Could you check a few things on this model? Use its own coordinates, in mm. A direction names the side the tool comes from. Give positions to 0.01 mm unless a question says otherwise; leave off trailing zeros. Write each loop counter-clockwise with the first axis right and the second up, starting at its lowest first coordinate (ties: lowest second). Pieces come first, ordered by that corner, then holes. Notation, with made-up numbers: (73.25, 74) - (109.25, 74) arc R33 cw to (109.25, 105) - close; hole circle Ø10 at (29.5, 23). An arc over 180 degrees is marked (long way). Answer as CSV lines item,"result". Start each with the question number.
Q1. Will these pins go through, and if not, where does the flat tip stop? pin 1 Ø10 at (x, y) = (-63.5, -2.5) entering from +Z; pin 2 Ø3.5 at (x, y) = (-33.73, -1.13) entering from -Z; pin 3 Ø2 at (y, z) = (13.87, 20.1) entering from -X.
Q2. Imagine slicing it at B-B on z = 3. List the corners of the cut face in (x, y) for me.
Q3. Imagine slicing it at C-C on y = 7. List the corners of the cut face in (x, z) for me, and give its area (3 significant figures).
Q4. On a 3-axis mill with a long thin cutter (end or side, diameter ignored), from which of +Z, -Z, +X, -X, +Y, -Y can I reach the whole of each face in a straight line? I mean faces 4 (the face through (-36, -5.5, 16)), 5 (the face through (-42.045, -7.086, 16.628)), 6 (the face through (-34, 10, 6.7)), 7 (the face through (-34.34, 23.97, 12.44)), 8 (the face through (-32.567, 14, 10)). Say none if no direction works.
Q5. If I drill on line 1 along Z through (x, y) = (-31.4, 3.87); line 2 along Y through (x, z) = (-51, 6); line 3 along Z through (x, y) = (-47, 7), over which ranges is the centre line in solid material (lowest first)?
Q6. Imagine slicing it at D-D on z = 17.5. List the corners of the cut face in (x, y) for me.
Q7. Imagine slicing it at A-A on x = -52. List the corners of the cut face in (y, z) for me.
Q8. We'd pull the mould along Y, two halves only. Please class faces 1 (the face through (-31.071, -4.074, 15.968)), 2 (the face through (-29.567, 13, 15)), 3 (the face through (-32.567, 14, 20)): pulls with the +Y half, pulls with the -Y half, needs draft (parallel to the pull), parting line crosses it, or undercut.
```python
from build123d import *

# Parameters (mm, degrees)
SKETCH_1_R                = 1.5
SKETCH_1_R_2              = 6.25
EXTRUDE_1_DEPTH           = 25.5
SKETCH_2_R                = 18.5
CUT_EXTRUDE_1_DEPTH       = 17.5
SKETCH_3_W                = 9.3
SKETCH_3_H                = 31.5
CUT_EXTRUDE_2_DEPTH       = 6.7
FILLET_1_R                = 20
SKETCH_4_R                = 1.5
CUT_EXTRUDE_3_DEPTH       = 44.630787393
FILLET_3_R                = 2
FILLET_4_R                = 2
FILLET_5_R                = 5
SKETCH_5_R                = 6
CUT_EXTRUDE_4_DEPTH       = 4
SKETCH_6_R                = 1.3
CUT_EXTRUDE_5_DEPTH       = 3
MOVE_BODY_1_OUTLINE_R     = 1.5
MOVE_BODY_1_OUTLINE_R_2   = 6.25
MOVE_BODY_1_DEPTH         = 25.5
MOVE_START                = 6.7
MOVE_BODY_1_2_OUTLINE_R   = 1.5
MOVE_BODY_1_2_OUTLINE_R_2 = 18.5
MOVE_BODY_1_2_DEPTH       = 18.8
MOVE_BODY_1_3_OUTLINE_R   = 1.5
MOVE_BODY_1_3_OUTLINE_R_2 = 6.25
MOVE_BODY_1_3_DEPTH       = 8
MOVE_START_2              = -29.5669682
MOVE_BODY_1_4_OUTLINE_W   = 31.5
MOVE_BODY_1_4_OUTLINE_H   = 18.8
MOVE_BODY_1_4_DEPTH       = 9.2969682
MOVE_START_3              = -32.5669682
MOVE_BODY_1_5_OUTLINE_R   = 1.3
MOVE_BODY_1_5_DEPTH       = 3
MOVE_START_4              = -21
MOVE_BODY_1_6_DEPTH       = 47
MOVE_START_5              = 22
MOVE_BODY_1_7_OUTLINE_R   = 6
MOVE_BODY_1_7_DEPTH       = 4


with BuildPart() as part:
    # 草图1 → 凸台-拉伸1 (new body)
    with BuildSketch(Plane.XY):
        with BuildLine():
            Line((21, 0), (21, 26))
            Line((21, 26), (-29.5669682, 26))
            Line((-29.5669682, 26), (-29.5669682, -5.5))
            Line((-29.5669682, -5.5), (-20.2669682, -5.5))
            ThreePointArc((-20.2669682, -5.5), (2.774316836, -20.815935388), (21, 0))
        make_face()
        with Locations((15.5, 0)):
            Circle(SKETCH_1_R, mode=Mode.SUBTRACT)
        with Locations((-15.5, 0)):
            Circle(SKETCH_1_R, mode=Mode.SUBTRACT)
        with Locations((-7.75, 13.423393759)):
            Circle(SKETCH_1_R, mode=Mode.SUBTRACT)
        with Locations((7.75, 13.423393759)):
            Circle(SKETCH_1_R, mode=Mode.SUBTRACT)
        with Locations((7.75, -13.423393759)):
            Circle(SKETCH_1_R, mode=Mode.SUBTRACT)
        with Locations((-7.75, -13.423393759)):
            Circle(SKETCH_1_R, mode=Mode.SUBTRACT)
        with Locations((0, 7)):
            Circle(SKETCH_1_R_2, mode=Mode.SUBTRACT)
    extrude(amount=EXTRUDE_1_DEPTH)

    # 草图2 → 切除-拉伸1 (cut)
    with BuildSketch(Plane.XY.offset(25.5)):
        Circle(SKETCH_2_R)
    extrude(amount=-CUT_EXTRUDE_1_DEPTH, mode=Mode.SUBTRACT)

    # 草图3 → 切除-拉伸2 (cut)
    with BuildSketch(Plane(origin=(0, 0, 0), x_dir=(-1, 0, 0), z_dir=(0, 0, -1))):
        with Locations((24.92, 10.25)):
            Rectangle(SKETCH_3_W, SKETCH_3_H)
    extrude(amount=-CUT_EXTRUDE_2_DEPTH, mode=Mode.SUBTRACT)

    # 圆角1
    fillet_1_edges = [part.edges().sort_by_distance(p)[0] for p in [
        (21, 26, 12.75),
    ]]
    fillet(fillet_1_edges, radius=FILLET_1_R)

    # 草图4 → 切除-拉伸3 (cut, through all)
    with BuildSketch(Plane(origin=(0, 0, 6.7), x_dir=(-1, 0, 0), z_dir=(0, 0, -1))):
        with Locations((25.407304845, 18.87)):
            Circle(SKETCH_4_R)
        with Locations((25.407304845, -1.13)):
            Circle(SKETCH_4_R)
    extrude(amount=-CUT_EXTRUDE_3_DEPTH, mode=Mode.SUBTRACT)

    # 圆角3
    fillet_3_edges = [part.edges().sort_by_distance(p)[0] for p in [
        (-29.5669682, 10.25, 25.5),
    ]]
    fillet(fillet_3_edges, radius=FILLET_3_R)

    # 圆角4
    fillet_4_edges = [part.edges().sort_by_distance(p)[0] for p in [
        (-20.2669682, -5.5, 12.75),
    ]]
    fillet(fillet_4_edges, radius=FILLET_4_R)

    # 圆角5
    # the kernel refuses this fillet: 5 mm, written as the material it takes off along each edge
    with BuildSketch(Plane(origin=(-29.5669682, -5.5, -5.8), x_dir=(1, 0, 0), z_dir=(0, 0, 1))) as fillet_5_piece_1:
        with BuildLine():
            CenterArc((FILLET_5_R, FILLET_5_R), FILLET_5_R, 180, 90)
            Line((0, FILLET_5_R), (0, 0))
            Line((0, 0), (FILLET_5_R, 0))
        make_face()
    extrude(amount=41.8, mode=Mode.SUBTRACT)

    # 草图5 → 切除-拉伸4 (cut)
    with BuildSketch(Plane(origin=(0, 26, 0), x_dir=(1, 0, 0), z_dir=(0, 1, 0))):
        with Locations(Location((-21.5669682, -17.5, 0), (0, 0, 270))):
            Circle(SKETCH_5_R)
    extrude(amount=-CUT_EXTRUDE_4_DEPTH, mode=Mode.SUBTRACT)

    # 草图6 → 切除-拉伸5 (cut)
    with BuildSketch(Plane.ZY.offset(29.5669682)):
        with Locations(Location((20.1, 13.87, 0), (0, 0, 270))):
            Circle(SKETCH_6_R)
        with Locations(Location((20.1, 3.87, 0), (0, 0, 270))):
            Circle(SKETCH_6_R)
        with Locations(Location((10.1, 3.87, 0), (0, 0, 270))):
            Circle(SKETCH_6_R)
        with Locations(Location((10.1, 13.87, 0), (0, 0, 270))):
            Circle(SKETCH_6_R)
    extrude(amount=-CUT_EXTRUDE_5_DEPTH, mode=Mode.SUBTRACT)

    # Move Body 1: read off the stored shape, not the designer's step
    # Move Body 1 outline → Move Body 1 (cut)
    with BuildSketch(Plane.XY):
        with BuildLine():
            Line((1, 26), (-20.27, 26))
            Line((-20.27, 26), (-20.27, 22))
            Line((-20.27, 22), (-20.27, -6.146923411))
            ThreePointArc((-20.27, -6.146923411), (-20.024941251, -6.475836873), (-19.852135348, -6.847826087))
            ThreePointArc((-19.852135348, -6.847826087), (3.471682423, -20.711045873), (21, 0))
            Line((21, 0), (21, 6))
            ThreePointArc((21, 6), (15.142135624, 20.142135624), (1, 26))
        make_face()
        with Locations((7.75, 13.423393759)):
            Circle(MOVE_BODY_1_OUTLINE_R, mode=Mode.SUBTRACT)
        with Locations((-7.75, -13.423393759)):
            Circle(MOVE_BODY_1_OUTLINE_R, mode=Mode.SUBTRACT)
        with Locations((7.75, -13.423393759)):
            Circle(MOVE_BODY_1_OUTLINE_R, mode=Mode.SUBTRACT)
        with Locations((-15.5, 0)):
            Circle(MOVE_BODY_1_OUTLINE_R, mode=Mode.SUBTRACT)
        with Locations((15.5, 0)):
            Circle(MOVE_BODY_1_OUTLINE_R, mode=Mode.SUBTRACT)
        with Locations((-7.75, 13.423393759)):
            Circle(MOVE_BODY_1_OUTLINE_R, mode=Mode.SUBTRACT)
        with Locations((0, 7)):
            Circle(MOVE_BODY_1_OUTLINE_R_2, mode=Mode.SUBTRACT)
    extrude(amount=MOVE_BODY_1_DEPTH, mode=Mode.SUBTRACT)

    # Move Body 1 2 outline → Move Body 1 2 (add)
    with BuildSketch(Plane.XY.offset(MOVE_START)):
        with BuildLine():
            Line((-20.27, 26), (-60.133936399, 26))
            ThreePointArc((-60.133936399, 26), (-74.276072023, 20.142135624), (-80.133936399, 6))
            Line((-80.133936399, 6), (-80.133936399, 0))
            ThreePointArc((-80.133936399, 0), (-62.605618822, -20.711045873), (-39.281801051, -6.847826087))
            ThreePointArc((-39.281801051, -6.847826087), (-38.552080618, -5.871450365), (-37.391121494, -5.5))
            Line((-37.391121494, -5.5), (-34.5669682, -5.5))
            ThreePointArc((-34.5669682, -5.5), (-31.031434294, -4.035533906), (-29.5669682, -0.5))
            ThreePointArc((-29.5669682, -0.5), (-28.102502106, -4.035533905), (-24.5669682, -5.5))
            Line((-24.5669682, -5.5), (-21.742814905, -5.5))
            ThreePointArc((-21.742814905, -5.5), (-20.938499413, -5.668859211), (-20.27, -6.146923411))
            Line((-20.27, -6.146923411), (-20.27, 22))
            Line((-20.27, 22), (-20.27, 26))
        make_face()
        with Locations((-33.726631554, -1.13)):
            Circle(MOVE_BODY_1_2_OUTLINE_R, mode=Mode.SUBTRACT)
        with Locations((-25.407304845, -1.13)):
            Circle(MOVE_BODY_1_2_OUTLINE_R, mode=Mode.SUBTRACT)
        with Locations((-33.726631554, 18.87)):
            Circle(MOVE_BODY_1_2_OUTLINE_R, mode=Mode.SUBTRACT)
        with Locations((-25.407304845, 18.87)):
            Circle(MOVE_BODY_1_2_OUTLINE_R, mode=Mode.SUBTRACT)
        with Locations((-59.133936399, 0)):
            Circle(MOVE_BODY_1_2_OUTLINE_R_2, mode=Mode.SUBTRACT)
    extrude(amount=MOVE_BODY_1_2_DEPTH)

    # Move Body 1 3 outline → Move Body 1 3 (add)
    with BuildSketch(Plane.XY):
        with BuildLine():
            Line((-38.863936399, 22), (-38.863936399, 26))
            Line((-38.863936399, 26), (-60.133936399, 26))
            ThreePointArc((-60.133936399, 26), (-74.276072023, 20.142135624), (-80.133936399, 6))
            Line((-80.133936399, 6), (-80.133936399, 0))
            ThreePointArc((-80.133936399, 0), (-62.605618822, -20.711045873), (-39.281801051, -6.847826087))
            ThreePointArc((-39.281801051, -6.847826087), (-39.108995148, -6.475836873), (-38.863936399, -6.146923411))
            Line((-38.863936399, -6.146923411), (-38.863936399, 22))
        make_face()
        with Locations((-51.383936399, 13.423393759)):
            Circle(MOVE_BODY_1_3_OUTLINE_R, mode=Mode.SUBTRACT)
        with Locations((-66.883936399, -13.423393759)):
            Circle(MOVE_BODY_1_3_OUTLINE_R, mode=Mode.SUBTRACT)
        with Locations((-51.383936399, -13.423393759)):
            Circle(MOVE_BODY_1_3_OUTLINE_R, mode=Mode.SUBTRACT)
        with Locations((-74.633936399, 0)):
            Circle(MOVE_BODY_1_3_OUTLINE_R, mode=Mode.SUBTRACT)
        with Locations((-43.633936399, 0)):
            Circle(MOVE_BODY_1_3_OUTLINE_R, mode=Mode.SUBTRACT)
        with Locations((-59.133936399, 7)):
            Circle(MOVE_BODY_1_3_OUTLINE_R_2, mode=Mode.SUBTRACT)
        with Locations((-66.883936399, 13.423393759)):
            Circle(MOVE_BODY_1_3_OUTLINE_R, mode=Mode.SUBTRACT)
    extrude(amount=MOVE_BODY_1_3_DEPTH)

    # Move Body 1 4 outline → Move Body 1 4 (cut)
    with BuildSketch(Plane.YZ.offset(MOVE_START_2)):
        with Locations((10.25, 16.1)):
            Rectangle(MOVE_BODY_1_4_OUTLINE_W, MOVE_BODY_1_4_OUTLINE_H)
    extrude(amount=MOVE_BODY_1_4_DEPTH, mode=Mode.SUBTRACT)

    # Move Body 1 5 outline → Move Body 1 5 (cut)
    with BuildSketch(Plane.YZ.offset(MOVE_START_3)):
        with Locations((13.87, 20.1)):
            Circle(MOVE_BODY_1_5_OUTLINE_R)
        with Locations((3.87, 20.1)):
            Circle(MOVE_BODY_1_5_OUTLINE_R)
        with Locations((3.87, 10.1)):
            Circle(MOVE_BODY_1_5_OUTLINE_R)
        with Locations((13.87, 10.1)):
            Circle(MOVE_BODY_1_5_OUTLINE_R)
    extrude(amount=MOVE_BODY_1_5_DEPTH, mode=Mode.SUBTRACT)

    # Move Body 1 6 outline → Move Body 1 6 (cut)
    with BuildSketch(Plane(origin=(0, 0, 0), x_dir=(1, 0, 0), z_dir=(0, 1, 0)).offset(MOVE_START_4)):
        with BuildLine():
            ThreePointArc((-29.5669682, -23.5), (-30.152754638, -24.914213563), (-31.5669682, -25.5))
            Line((-31.5669682, -25.5), (-20.27, -25.5))
            Line((-20.27, -25.5), (-20.27, -6.7))
            Line((-20.27, -6.7), (-29.566968204, -6.7))
            Line((-29.566968204, -6.7), (-29.5669682, -23.5))
        make_face()
    extrude(amount=MOVE_BODY_1_6_DEPTH, mode=Mode.SUBTRACT)

    # Move Body 1 7 outline → Move Body 1 7 (cut)
    with BuildSketch(Plane(origin=(0, 0, 0), x_dir=(1, 0, 0), z_dir=(0, 1, 0)).offset(MOVE_START_5)):
        with Locations((-37.5669682, -17.5)):
            Circle(MOVE_BODY_1_7_OUTLINE_R)
    extrude(amount=MOVE_BODY_1_7_DEPTH, mode=Mode.SUBTRACT)


solid = part.part
```
Conclusion:
1,pin 1,"z = 8"
1,pin 2,"z = 6.7"
1,pin 3,"x = -78.92"
2,outline,"(-80.13, 0) arc R21 ccw to (-39.28, -6.85) arc R2 cw to (-38.86, -6.15) - (-38.86, 26) - (-60.13, 26) arc R20 ccw to (-80.13, 6) - close; hole circle Ø3 at (-74.63, 0); hole circle Ø3 at (-66.88, -13.42); hole circle Ø3 at (-66.88, 13.42); hole circle Ø12.5 at (-59.13, 7); hole circle Ø3 at (-51.38, -13.42); hole circle Ø3 at (-51.38, 13.42); hole circle Ø3 at (-43.63, 0)"
3,outline,"(-80.11, 0) - (-65.38, 0) - (-65.38, 8) - (-76.26, 8) - (-76.26, 25.5) - (-80.11, 25.5) - close; (-52.88, 0) - (-38.86, 0) - (-38.86, 6.7) - (-29.57, 6.7) - (-29.57, 23.5) arc R2 ccw to (-31.57, 25.5) - (-42.01, 25.5) - (-42.01, 8) - (-52.88, 8) - close"
3,area,"526 mm^2"
4,face 4,"+Z, -Z, +X, -Y"
4,face 5,"+Z"
4,face 6,"-Z, +X, +Y, -Y"
4,face 7,"+Y"
4,face 8,"+X"
5,line 1,"6.7 to 8.8, 11.4 to 18.8, 21.4 to 25.49"
5,line 2,"-19.36 to -14.87, -11.97 to 11.97, 14.87 to 26"
5,line 3,"0 to 8"
6,outline,"(-80.13, 0) arc R21 ccw to (-39.28, -6.85) arc R2 cw to (-37.39, -5.5) - (-34.57, -5.5) arc R5 ccw to (-29.57, -0.5) - (-29.57, 26) - (-31.57, 26) - (-31.57, 22) - (-43.57, 22) - (-43.57, 26) - (-60.13, 26) arc R20 ccw to (-80.13, 6) - close; hole circle Ø37 at (-59.13, 0); hole circle Ø3 at (-33.73, -1.13); hole circle Ø3 at (-33.73, 18.87)"
7,outline,"(-19.75, 0) - (-14.79, 0) - (-14.79, 8) - (-17.07, 8) - (-17.07, 25.5) - (-19.75, 25.5) - close; (-12.06, 0) - (12.06, 0) - (12.06, 8) - (-12.06, 8) - close; (14.79, 0) - (26, 0) - (26, 25.5) - (17.07, 25.5) - (17.07, 8) - (14.79, 8) - close"
8,face 1,"pulls with the -Y half"
8,face 2,"needs draft"
8,face 3,"undercut"
